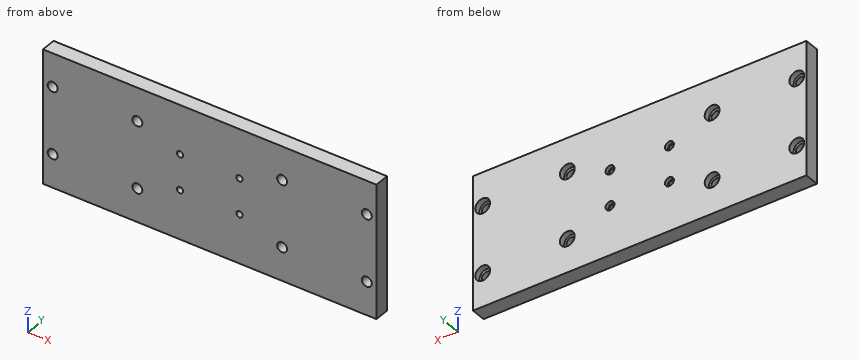
```python
from build123d import *

# Parameters (mm, degrees)
CROQUIS1_W              = 224.48
CROQUIS1_H              = 90
SALIENTE_EXTRUIR1_DEPTH = 10
CROQUIS2_R              = 3.35
CORTAR_EXTRUIR1_DEPTH   = 11
CROQUIS22_R             = 2.1
CORTAR_EXTRUIR3_DEPTH   = 11
CROQUIS25_R             = 5
CORTAR_EXTRUIR4_DEPTH   = 4
CROQUIS26_R             = 3
CORTAR_EXTRUIR5_DEPTH   = 2.5
CROQUIS27_R             = 3.35
CORTAR_EXTRUIR6_DEPTH   = 11
CROQUIS28_R             = 5
CORTAR_EXTRUIR7_DEPTH   = 4


with BuildPart() as part:
    # Croquis1 → Saliente-Extruir1 (new body)
    with BuildSketch(Plane(origin=(0, 0, 0), x_dir=(1, 0, 0), z_dir=(0, 1, 0))):
        Rectangle(CROQUIS1_W, CROQUIS1_H)
    extrude(amount=SALIENTE_EXTRUIR1_DEPTH)

    # Croquis2 → Cortar-Extruir1 (cut, through all)
    with BuildSketch(Plane(origin=(0, 0, 0), x_dir=(1, 0, 0), z_dir=(0, 1, 0))):
        with Locations((-105.74, 22.5)):
            Circle(CROQUIS2_R)
        with Locations((105.74, 22.5)):
            Circle(CROQUIS2_R)
        with Locations((105.74, -22.5)):
            Circle(CROQUIS2_R)
        with Locations((-105.74, -22.5)):
            Circle(CROQUIS2_R)
    extrude(amount=CORTAR_EXTRUIR1_DEPTH, mode=Mode.SUBTRACT)

    # Croquis22 → Cortar-Extruir3 (cut, through all)
    with BuildSketch(Plane(origin=(0, 0, 0), x_dir=(1, 0, 0), z_dir=(0, 1, 0))):
        with Locations((20, 12)):
            Circle(CROQUIS22_R)
        with Locations((-20, 12)):
            Circle(CROQUIS22_R)
        with Locations((-20, -12)):
            Circle(CROQUIS22_R)
        with Locations((20, -12)):
            Circle(CROQUIS22_R)
    extrude(amount=CORTAR_EXTRUIR3_DEPTH, mode=Mode.SUBTRACT)

    # Croquis25 → Cortar-Extruir4 (cut)
    with BuildSketch(Plane(origin=(0, 10, 0), x_dir=(1, 0, 0), z_dir=(0, 1, 0))):
        with Locations((-105.74, 22.5)):
            Circle(CROQUIS25_R)
        with Locations((-105.74, -22.5)):
            Circle(CROQUIS25_R)
        with Locations((105.74, 22.5)):
            Circle(CROQUIS25_R)
        with Locations((105.74, -22.5)):
            Circle(CROQUIS25_R)
    extrude(amount=-CORTAR_EXTRUIR4_DEPTH, mode=Mode.SUBTRACT)

    # Croquis26 → Cortar-Extruir5 (cut)
    with BuildSketch(Plane(origin=(0, 10, 0), x_dir=(1, 0, 0), z_dir=(0, 1, 0))):
        with Locations((-20, 12)):
            Circle(CROQUIS26_R)
        with Locations((20, 12)):
            Circle(CROQUIS26_R)
        with Locations((20, -12)):
            Circle(CROQUIS26_R)
        with Locations((-20, -12)):
            Circle(CROQUIS26_R)
    extrude(amount=-CORTAR_EXTRUIR5_DEPTH, mode=Mode.SUBTRACT)

    # Croquis27 → Cortar-Extruir6 (cut, through all)
    with BuildSketch(Plane(origin=(0, 10, 0), x_dir=(1, 0, 0), z_dir=(0, 1, 0))):
        with Locations((-48.74, 22.5)):
            Circle(CROQUIS27_R)
        with Locations((48.74, 22.5)):
            Circle(CROQUIS27_R)
        with Locations((48.74, -22.5)):
            Circle(CROQUIS27_R)
        with Locations((-48.74, -22.5)):
            Circle(CROQUIS27_R)
    extrude(amount=-CORTAR_EXTRUIR6_DEPTH, mode=Mode.SUBTRACT)

    # Croquis28 → Cortar-Extruir7 (cut)
    with BuildSketch(Plane(origin=(0, 10, 0), x_dir=(1, 0, 0), z_dir=(0, 1, 0))):
        with Locations((-48.74, 22.5)):
            Circle(CROQUIS28_R)
        with Locations((-48.74, -22.5)):
            Circle(CROQUIS28_R)
        with Locations((48.74, -22.5)):
            Circle(CROQUIS28_R)
        with Locations((48.74, 22.5)):
            Circle(CROQUIS28_R)
    extrude(amount=-CORTAR_EXTRUIR7_DEPTH, mode=Mode.SUBTRACT)


solid = part.part
```
Model file for the job. Use its own axes, mm. Coordinates: 2 decimals unless noted, no trailing zeros. Loops run counter-clockwise (first coordinate to the right, second up) from the corner with the lowest first, then second, coordinate; pieces in that order, holes last. Notation, with made-up numbers: (19.5, 78) - (28.5, 78) arc R23 ccw to (28.5, 100) - close; hole circle Ø8 at (-12, 82). An arc over 180 degrees is marked (long way). Write item = value, one per line. Start each with the question number.
Item 1: Saw through at C-C, the plane z = -22.5. State how many separate pieces and enclosed holes the cut face has, then the cut area to 3 significant figures.
Item 2: Drop flat-ended pins along their axis: pin 1 Ø5.5 at (x, z) = (-20, 12) entering from +Y; pin 2 Ø8 at (x, z) = (48.74, -22.5) entering from +Y. Give the stop position or say it passes through.
Item 3: Saw through at A-A, the plane z = 12. List the corners of the cut face in (x, y), then the cut area to 3 significant figures.
Item 4: Wall check: probe 1 along X at (y, z) = (2.5, -12); probe 2 along Z at (x, y) = (49, 2); probe 3 along Z at (x, y) = (48.74, 8.6). Give the ranges that are in metal, low to high. Write a range as [from, to].
Item 5: Saw through at B-B, the plane x = -105.74. List the corners of the cut face in (y, z).
Answers:
q1.separate_pieces = 5
q1.enclosed_holes = 0
q1.area = 1,920 mm2
q2.pin_1 = 7.5
q2.pin_2 = 6
q3.outline = (-112.24, 0) - (-22.1, 0) - (-22.1, 7.5) - (-23, 7.5) - (-23, 10) - (-112.24, 10) - close; (-17.9, 0) - (17.9, 0) - (17.9, 7.5) - (17, 7.5) - (17, 10) - (-17, 10) - (-17, 7.5) - (-17.9, 7.5) - close; (22.1, 0) - (112.24, 0) - (112.24, 10) - (23, 10) - (23, 7.5) - (22.1, 7.5) - close
q3.area = 2,150 mm2
q4.probe_1 = [-112.24, -22.1], [-17.9, 17.9], [22.1, 112.24]
q4.probe_2 = [-45, -25.84], [-19.16, 19.16], [25.84, 45]
q4.probe_3 = [-45, -27.5], [-17.5, 17.5], [27.5, 45]
q5.outline = (0, -45) - (10, -45) - (10, -27.5) - (6, -27.5) - (6, -25.85) - (0, -25.85) - close; (0, -19.15) - (6, -19.15) - (6, -17.5) - (10, -17.5) - (10, 17.5) - (6, 17.5) - (6, 19.15) - (0, 19.15) - close; (0, 25.85) - (6, 25.85) - (6, 27.5) - (10, 27.5) - (10, 45) - (0, 45) - close
